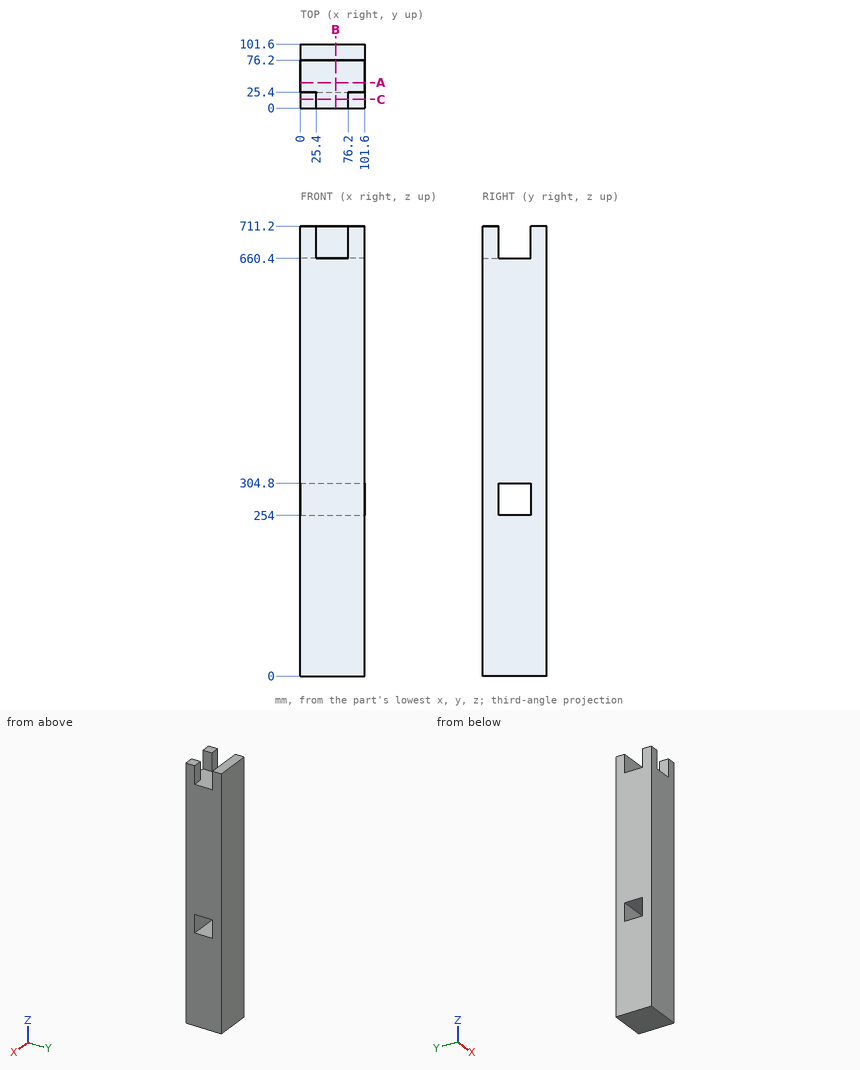
Print and shaded views of the part. All mm, measured from the part's lowest x, y and z. Coordinates: 2 decimals unless noted, no trailing zeros. Order: outer loops, then holes, each group sorted by start corner. A loop starts at its lowest first (then second) coordinate and runs counter-clockwise, first axis right, second up. Notation, with made-up numbers: M 51,43.5 L 107,43.5 A31 ccw 107,79.5 Z; hole C -39.5,51 d10. An arc over 180 degrees is marked long. Write each question's results on one line, items separated by ' | '. Start each with the question number.
Q1. Flat gauge pin, fed straight in: P1, Ø12, axis at x = 47, y = 43, coming from the +Z side. Where does the tip first touch, or does it go through?
Q2. Drill centre lines: probe 1 along Z at (x, y) = (73, 46); probe 2 along Y at (x, z) = (35.5, 298); probe 3 along Z at (x, y) = (29.5, 6). Where is each one in solid material? Low to high. Write a range as from..to.
Q3. Cut at C-C (y = 14). List the corners of the cut face in (x, z), then the cut area to 3 significant figures.
Q4. Cut at B-B (x = 56). List the corners of the cut face in (y, z).
Q5. Cut at A-A (y = 40.5). List the corners of the cut face in (x, z).
Found:
1) P1: z = 660.4
2) probe 1: 0..254, 304.8..660.4 | probe 2: 0..25.4, 76.2..101.6 | probe 3: 0..660.4
3) outline: M 0,0 L 101.6,0 L 101.6,711.2 L 76.2,711.2 L 76.2,660.4 L 25.4,660.4 L 25.4,711.2 L 0,711.2 Z | area: 69,700 mm²
4) outline: M 0,0 L 101.6,0 L 101.6,711.2 L 76.2,711.2 L 76.2,660.4 L 0,660.4 Z; hole M 25.4,254 L 76.2,254 L 76.2,304.8 L 25.4,304.8 Z
5) outline: M 0,0 L 101.6,0 L 101.6,254 L 0,254 Z; M 0,304.8 L 101.6,304.8 L 101.6,660.4 L 0,660.4 Z
